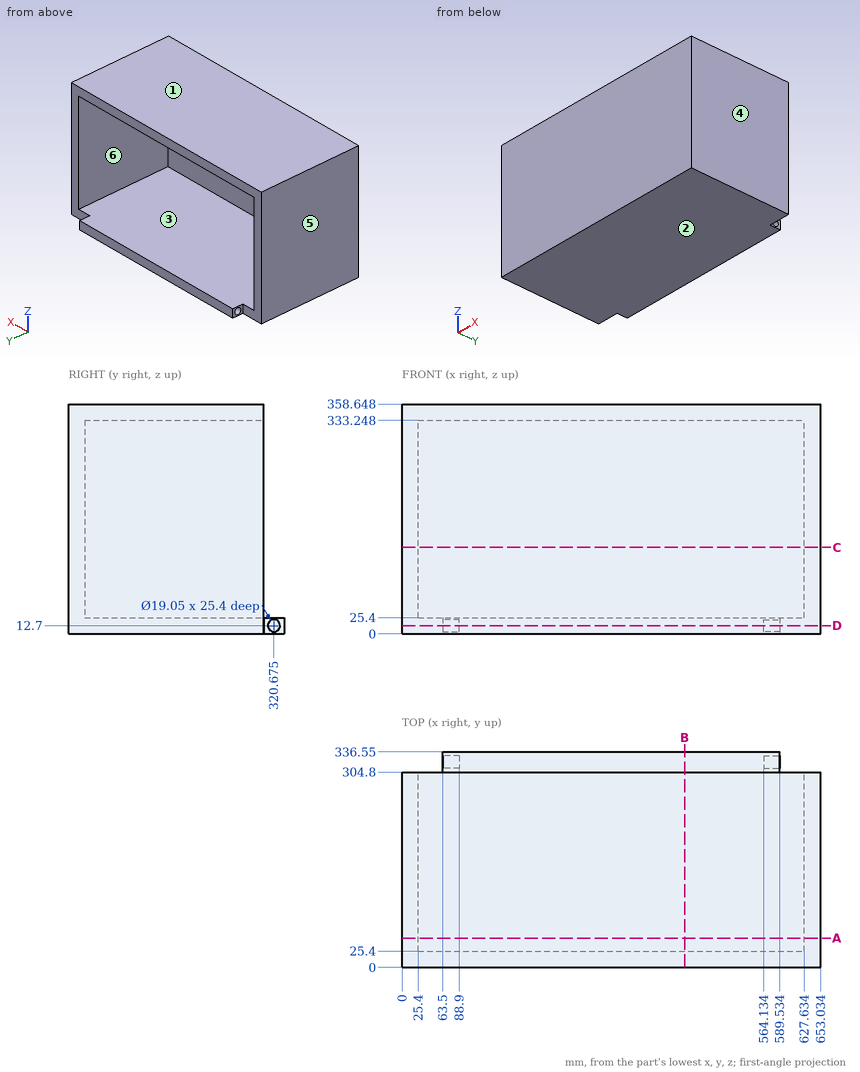
Here's the drawing with two shaded views (mm, measured from the low corner). I have some questions. A direction names the side the tool comes from. Coordinates: 2 decimals unless noted, no trailing zeros. Order: outer loops, then holes, each group sorted by start corner. A loop starts at its lowest first (then second) coordinate and runs counter-clockwise, first axis right, second up.
Q1. Suppose I cut it at A-A on y = 45.5. Please give me the cut outline in (x, z).
Q2. Suppose I cut it at D-D on z = 12.7. Please give me the cut outline in (x, y), and give its area (3 significant figures).
Q3. Which directions (+Z, -Z, +X, -X, +Y, -Y) give clear straight access to the entire face, cutting with the end or side of a thin tool? Please do the marked faces 5 and 6.
Q4. Thinking about a two-plate mould opening in Z: for the marked faces 1, 2, 3 and 4, which applies, released by +Z, released by -Z, zero draft, split by the parting line, or undercut?
Q5. Will these pins go through, and if not, where does the flat tip stop? pin 1 (9.5 mm diameter, centred on y = 323.5, z = 14.5, fed in from -X); pin 2 (15 mm diameter, centred on y = 320.675, z = 12.7, fed in from +X); pin 3 (10 mm diameter, centred on x = 561.5, z = 268.5, fed in from +Y).
Q6. Suppose I cut it at C-C on z = 135. Please give me the cut outline in (x, y).
Q7. Suppose I cut it at B-B on x = 441. Please give me the cut outline in (y, z), and give its area (3 significant figures).
Q8. Please list where these lines run through material, in increasing order: L1, parallel to Z at x = 127, y = 40.5; L2, parallel to Y at x = 80.75, z = 12.7; L3, parallel to X at y = 116.5, z = 178.
Answer:
1. outline: (0, 0) - (653.03, 0) - (653.03, 358.65) - (0, 358.65) - close; hole (25.4, 25.4) - (627.63, 25.4) - (627.63, 333.25) - (25.4, 333.25) - close
2. outline: (0, 0) - (653.03, 0) - (653.03, 304.8) - (589.53, 304.8) - (589.53, 311.15) - (564.13, 311.15) - (564.13, 330.2) - (589.53, 330.2) - (589.53, 336.55) - (63.5, 336.55) - (63.5, 330.2) - (88.9, 330.2) - (88.9, 311.15) - (63.5, 311.15) - (63.5, 304.8) - (0, 304.8) - close
2. area: 215,000 mm2
3. face 5: +Z, -Z, -X, +Y, -Y
3. face 6: +Y
4. face 1: released by +Z
4. face 2: released by -Z
4. face 3: undercut
4. face 4: zero draft
5. pin 1: stops at x = 88.9
5. pin 2: stops at x = 564.13
5. pin 3: stops at y = 25.4
6. outline: (0, 0) - (653.03, 0) - (653.03, 304.8) - (627.63, 304.8) - (627.63, 25.4) - (25.4, 25.4) - (25.4, 304.8) - (0, 304.8) - close
7. outline: (0, 0) - (336.55, 0) - (336.55, 25.4) - (25.4, 25.4) - (25.4, 333.25) - (304.8, 333.25) - (304.8, 358.65) - (0, 358.65) - close
7. area: 24,100 mm2
8. L1: z = 0 to 25.4, 333.25 to 358.65
8. L2: y = 0 to 311.15, 330.2 to 336.55
8. L3: x = 0 to 25.4, 627.63 to 653.03
